Check sheet for the modelled part. Datum: model origin and axes. Units: mm. A direction names the side the tool comes from. Round coordinates to 2 decimals unless told otherwise and drop trailing zeros. Loops run counter-clockwise (first coordinate to the right, second up) from the corner with the lowest first, then second, coordinate; pieces in that order, holes last. Notation, with made-up numbers: (-23, 71) -> (1, 71) arc R12 ccw to (1, 77) -> close; hole circle Ø4 at (60.25, -25). An arc over 180 degrees is marked (long way). Use one line per item in the form item = value. Start each with the question number.
(1) Draft check along Z on faces 3 (the flat face through (-15, 6, -7)), 4 (the flat face through (-22, 6, 0)), 5 (the cylindrical face through (-7.05, 9.97, 10.42)). Enter one of: released by +Z, released by -Z, zero draft, split by the parting line, or undercut.
(2) Set-up check for faces 1 (the flat face through (0, 6, 0)), 2 (the cylindrical face through (-6.84, 3.94, 4.36)): record each of +Z, -Z, +X, -X, +Y, -Y from which the full face is reachable in a straight line by a thin tool's end or side.
(3) Sectioned sample at A-A (y = 6.75). Record the cut outline in (x, z), and give its area (3 significant figures).
(4) Material ranges on probe 1 along Z at (x, y) = (-23, 10.5); probe 2 along X at (y, z) = (1.75, -1.75); probe 3 along X at (y, z) = (10.5, 10.75), recorded low to high. Write a range as [from, to].
(5) Sectioned sample at D-D (y = 10.75). Record the cut outline in (x, z).
(6) Go/stop test with flat-tipped pins: pin 1 (3 mm diameter, centred on y = 8, z = -7, fed in from +X); pin 2 (1.5 mm diameter, centred on y = 2, z = -5, fed in from -X); pin 3 (6 mm diameter, centred on x = -22.5, y = 1.5, fed in from -Z); pin 4 (8 mm diameter, centred on x = -5.758, z = 9.242, fed in from -Y). Record where each tip stops, or that it passes through.
(7) Sectioned sample at B-B (z = 12). Record the cut outline in (x, y), and give its area (3 significant figures).
(8) Sectioned sample at C-C (x = -10). Record the cut outline in (y, z).
Autodesk Inventor part; units mm, degrees
ref_plane "YZ Plane" through (0, 0, 0) normal (1, 0, 0) x (0, 1, 0)
ref_plane "XZ Plane" through (0, 0, 0) normal (0, 1, 0) x (-1, 0, 0)
ref_plane "XY Plane" through (0, 0, 0) normal (0, 0, 1) x (1, 0, 0)
sketch "Szkic1" plane through (0, 0, 0) normal (0, 1, 0) x (-1, 0, 0)
  line L0 (0, 0) -> (30, 0)
  line L1 (30, 0) -> (30, 15)
  line L2 (30, 15) -> (0, 15)
  line L3 (0, 15) -> (0, 0)
  line L4 (0, 0) -> (15, 0)
  line L5 (15, 0) -> (15, -15)
  line L6 (15, -15) -> (0, -15)
  line L7 (0, -15) -> (0, 0)
  dimension "d0" = 30
  dimension "d1" = 15
  dimension "d2" = 15
  dimension "d3" = 15
extrude "Wyciągnięcie proste1" add sketch "Szkic1" along normal blind 12
sketch "Szkic2" plane through (0, 0, 0) normal (0, -1, 0) x (1, 0, 0)
  line L0 (0, 9.242) -> (-5.758, 9.242)
  line L1 (-30, 15) -> (0, 15)
  line L2 (-5.758, 15) -> (-5.758, 9.242)
  circle A0 centre (-5.758, 9.242) radius 5
  point P0 (0, 0)
  dimension "d6" = 5.758
  dimension "d7" = 5.758
  dimension "d8" = 10
extrude "Wyciągnięcie proste2" cut sketch "Szkic2" against normal blind 8
sketch "Szkic3" plane through (-5.758, 8, 9.242) normal (0, -1, 0) x (1, 0, 0)
  circle A0 centre (0, 0) radius 5
  circle A1 centre (0, 0) radius 1.75
  point P0 (5.758, -9.242)
  dimension "d11" = 3.5
extrude "Wyciągnięcie proste3" cut sketch "Szkic3" against normal blind 4 contours A1
thread "Gwint1"
properties part number "Footer"
Checks:
q1.face_3 = zero draft
q1.face_4 = released by -Z
q1.face_5 = undercut
q2.face_1 = +Z, -Z, +X, +Y, -Y
q2.face_2 = -Y
q3.outline = (-30, 0) -> (-15, 0) -> (-15, -15) -> (0, -15) -> (0, 15) -> (-30, 15) -> close; hole circle Ø10 at (-5.76, 9.24)
q3.area = 596 mm2
q4.probe_1 = [0, 15]
q4.probe_2 = [-15, 0]
q4.probe_3 = [-30, -6.65], [-4.87, 0]
q5.outline = (-30, 0) -> (-15, 0) -> (-15, -15) -> (0, -15) -> (0, 15) -> (-30, 15) -> close; hole circle Ø3.5 at (-5.76, 9.24)
q6.pin_1 = 0
q6.pin_2 = -15
q6.pin_3 = 0
q6.pin_4 = 8
q7.outline = (-30, 0) -> (-9.93, 0) -> (-9.93, 8) -> (-1.59, 8) -> (-1.59, 0) -> (0, 0) -> (0, 12) -> (-30, 12) -> close
q7.area = 293 mm2
q8.outline = (0, -15) -> (12, -15) -> (12, 15) -> (0, 15) -> (0, 11.89) -> (8, 11.89) -> (8, 6.6) -> (0, 6.6) -> close
